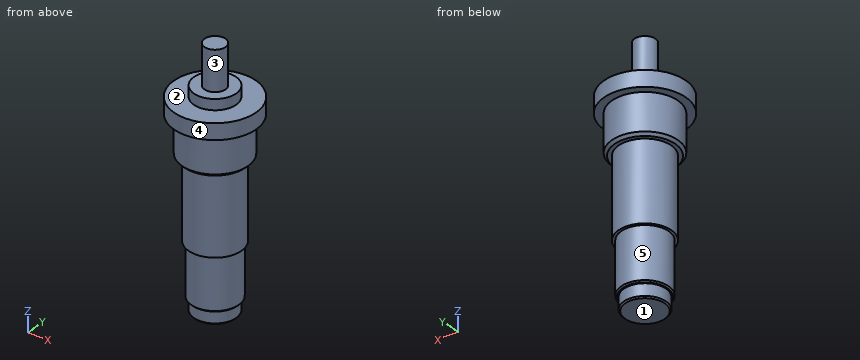
from build123d import *

# Parameters (mm, degrees)
CHAMFER_1_SIZE = 1
CHAMFER_2_SIZE = 0.5


with BuildPart() as part:
    # 草图1 → 旋转1 (revolve)
    with BuildSketch(Plane(origin=(0, 0, 0), x_dir=(0, 0, -1), z_dir=(1, 0, 0)), mode=Mode.PRIVATE) as revolve_1_sk:
        Polygon((-47.5, 0), (-47.5, 4), (-32.5, 4), (-32.5, 8), (-28.5, 8), (-28.5, 15.5), (-22.5, 15.5), (-22.5, 12.5), (-7.5, 12.5), (-7.5, 10), (22.5, 10), (22.5, 9), (42.5, 9), (42.5, 8), (47.5, 8), (47.5, 0), align=None)
    revolve(revolve_1_sk.sketch.rotate(Axis((0, 0, 113.714285714), (0, 0, -1)), 90), axis=Axis((0, 0, 113.714285714), (0, 0, -1)))

    # 倒角1
    chamfer_1_edges = [part.edges().sort_by_distance(p)[0] for p in [
        (-12.5, 0, 7.5),
    ]]
    chamfer(chamfer_1_edges, length=CHAMFER_1_SIZE)

    # 倒角2
    chamfer_2_edges = [part.edges().sort_by_distance(p)[0] for p in [
        (-8, 0, -47.5),
        (-9, 0, -42.5),
    ]]
    chamfer(chamfer_2_edges, length=CHAMFER_2_SIZE)


solid = part.part
CAD build for the part. Positions are in the model's coordinates, mm. Face numbers are marked on the shaded views. A direction names the side the tool comes from. Coordinates: 2 decimals unless noted, no trailing zeros. Loops run counter-clockwise (first coordinate to the right, second up) from the corner with the lowest first, then second, coordinate; pieces in that order, holes last. Notation, with made-up numbers: (-17.75, 62) - (4.25, 62) arc R11 ccw to (4.25, 72) - close; hole circle Ø2 at (-34, 78). An arc over 180 degrees is marked (long way). Write item = value, one per line. Start each with the question number.
Q1. Flat gauge pins, fed straight in: pin 1 Ø2 at (y, z) = (1.5, 5.5) entering from -X; pin 2 Ø1.5 at (x, y) = (12, 1) entering from +Z; pin 3 Ø1.5 at (x, z) = (-7.5, 0.5) entering from -Y. Where does each tip first touch, or does it go through?
Q2. Drill centre lines: L1, parallel to Z at x = -14, y = -2; L2, parallel to Y at x = -7.5, z = 8.5; L3, parallel to Z at x = 2, y = -3.5. Where is each one in solid material? Low to high.
Q3. Which spindle directions (+Z, -Z, +X, -X, +Y, -Y) get a long thin tool onto all of the face, cutting with end or side? Do the marked faces 4 and 5. Say none if no direction does.
Q4. Pull direction Z, two halves, no side cores. Call the marked faces 1, 2 and 3: pulls with the +Z half, pulls with the -Z half, needs draft (parallel to the pull), parting line crosses it, or undercut.
Q5. Cut at C-C, the plane z = -14.5. List the corners of the cut face in (x, y).
Q6. Cut at D-D, the plane z = 10.5. List the corners of the cut face in (x, y), then the cut area to 3 significant figures.
Computed:
q1.pin_1 = -9.99
q1.pin_2 = 28.5
q1.pin_3 = -7.38
q2.L1 = 22.5 to 28.5
q2.L2 = -10 to 10
q2.L3 = -47.5 to 32.5
q3.face_4 = +Z, -Z
q3.face_5 = -Z
q4.face_1 = pulls with the -Z half
q4.face_2 = pulls with the +Z half
q4.face_3 = needs draft
q5.outline = circle Ø20 at (0, 0)
q6.outline = circle Ø25 at (0, 0)
q6.area = 491 mm²
